Source: three-view drawing plus pictorial views. Frame: mm from the lowest corner of the part. Round coordinates to 2 decimals unless told otherwise and drop trailing zeros. Loops run counter-clockwise (first coordinate to the right, second up) from the corner with the lowest first, then second, coordinate; pieces in that order, holes last. Notation, with made-up numbers: (-2.5, 1.25) -> (4.5, 1.25) arc R31 ccw to (4.5, 38.25) -> close; hole circle Ø11 at (-29.5, -3.75). An arc over 180 degrees is marked (long way). One line per question, with ' | ' between items. Start each with the question number.
Q1. Contact query for flat-ended pins moving along their axis: P1, Ø1.5, axis at x = 82.5, z = 1.5, coming from the -Y side; P2, Ø1.5, axis at x = 85.5, y = 10, coming from the -Z side; P3, Ø0.5, axis at x = 9, z = 2.5, coming from the -Y side; P4, Ø1.5, axis at x = 73, z = 3, coming from the +Y side. Output: stop coordinate, or through.
Q2. Cut plane B-B on y = 4.5. Return loops of the section in (x, z).
Q3. Material intervals for L1, parallel to Z at x = 53.5, y = 10.75; L2, parallel to X at y = 5.25, z = 4.85; L3, parallel to X at y = 10.25, z = 3.2, sorted ascending.
Q4. Cut plane A-A on x = 20.5. Return loops of the section in (y, z).
Q5. Cut plane C-C on y = 10.5. Return loops of the section in (x, z), and give its area (3 significant figures).
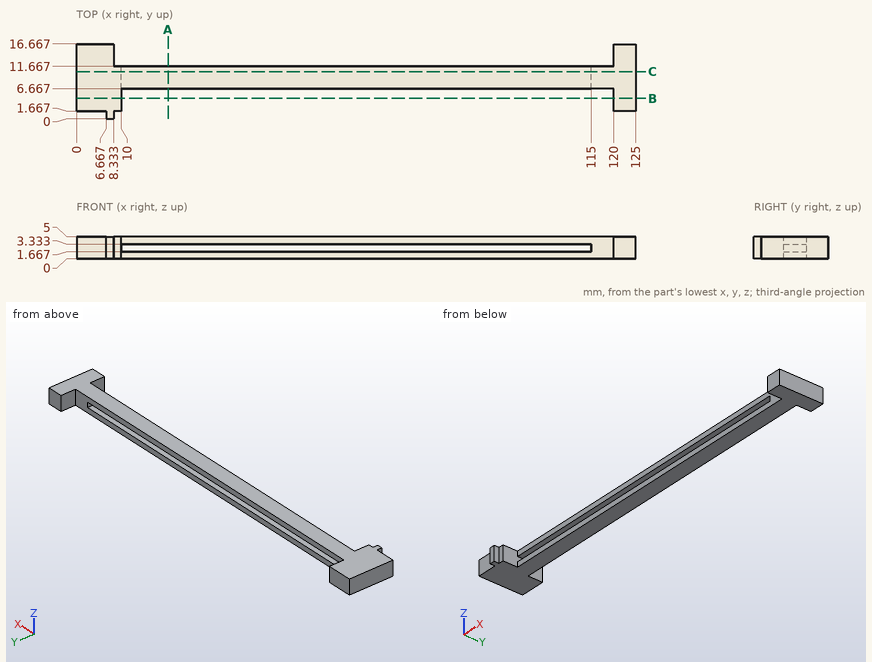
Results:
1) P1: y = 6.67 | P2: z = 0 | P3: y = 1.67 | P4: y = 11.67
2) outline: (0, 0) -> (10, 0) -> (10, 5) -> (0, 5) -> close; (120, 0) -> (125, 0) -> (125, 5) -> (120, 5) -> close
3) L1: 0 to 1.67, 3.33 to 5 | L2: 0 to 10, 120 to 125 | L3: 0 to 10, 115 to 125
4) outline: (6.67, 0) -> (11.67, 0) -> (11.67, 1.67) -> (6.67, 1.67) -> close; (6.67, 3.33) -> (11.67, 3.33) -> (11.67, 5) -> (6.67, 5) -> close
5) outline: (0, 0) -> (125, 0) -> (125, 5) -> (0, 5) -> close; hole (10, 1.67) -> (115, 1.67) -> (115, 3.33) -> (10, 3.33) -> close | area: 450 mm^2
